Geometry: final body of the model. Coordinates: model frame, mm. A direction names the side the tool comes from. Round coordinates to 2 decimals unless told otherwise and drop trailing zeros. Write each loop counter-clockwise with the first axis right and the second up, starting at its lowest first coordinate (ties: lowest second). Pieces come first, ordered by that corner, then holes. Notation, with made-up numbers: (27, -25) -> (65, -25) arc R36 cw to (65, 9) -> close; hole circle Ø9 at (38, 79). An arc over 180 degrees is marked (long way). Use one line per item in the form item = value. Start each with the question number.
1. Cut plane B-B, the plane y = 0. Return the cut outline in (x, z) (3 decimals).
2. Cut plane C-C, the plane x = 119. Return the cut outline in (y, z) (3 decimals), plus the area to 3 significant figures.
3. Cut plane A-A, the plane z = 18. Return the cut outline in (x, y) (3 decimals).
4. Pin query (flat end, axial travel): pin 1 Ø11.5 at (x, y) = (146.05, 0) entering from -Z. Return the tip coordinate at first contact, or that it passes through.
5. Line query: L1, parallel to X at y = 0, z = 23.55 (3 decimals); L2, parallel to Z at x = 103, y = 7.5 (3 decimals); L3, parallel to Y at x = 84, z = 13 (3 decimals). Output: solid intervals per line, ascending.
6. Cut plane D-D, the plane y = 7. Return the cut outline in (x, z) (3 decimals), plus the area to 3 significant figures.
7. Reachability of faces 4 (the face through (72, 12.7, 13)), 5 (the face through (74, -9.525, 13)) from +Z, -Z, +X, -X, +Y, -Y: full face, straight path, thin tool, end or side. Return the list, or none.
8. Draft query along Z for faces 1 (the face through (74, 0, 3.175)), 2 (the face through (72, 0, 25.4)), 3 (the face through (158.75, 11, 13)). Return one class per face: pulls with the +Z half, pulls with the -Z half, needs draft (parallel to the pull), parting line crosses it, or undercut.
```python
from build123d import *

# Parameters (mm, degrees)
SKETCH1_W           = 171.45
SKETCH1_H           = 25.4
SKETCH1_R           = 9.525
BOSS_EXTRUDE1_DEPTH = 25.4
SKETCH2_W           = 19.05
SKETCH2_H           = 19.05
CUT_EXTRUDE1_DEPTH  = 174.785938729


with BuildPart() as part:
    # Sketch1 → Boss-Extrude1 (new body)
    with BuildSketch(Plane.XY):
        with Locations((73.025, 0)):
            Rectangle(SKETCH1_W, SKETCH1_H)
        Circle(SKETCH1_R, mode=Mode.SUBTRACT)
        with Locations((146.05, 0)):
            Circle(SKETCH1_R, mode=Mode.SUBTRACT)
    extrude(amount=BOSS_EXTRUDE1_DEPTH)

    # Sketch2 → Cut-Extrude1 (cut, through all)
    with BuildSketch(Plane(origin=(158.75, 0, 0), x_dir=(0, 0, -1), z_dir=(1, 0, 0))):
        with Locations((-12.7, 0)):
            Rectangle(SKETCH2_W, SKETCH2_H)
    extrude(amount=-CUT_EXTRUDE1_DEPTH, mode=Mode.SUBTRACT)


solid = part.part
```
Outcome:
q1.outline = (-12.7, 0) -> (-9.525, 0) -> (-9.525, 3.175) -> (-12.7, 3.175) -> close; (-12.7, 22.225) -> (-9.525, 22.225) -> (-9.525, 25.4) -> (-12.7, 25.4) -> close; (9.525, 0) -> (136.525, 0) -> (136.525, 3.175) -> (9.525, 3.175) -> close; (9.525, 22.225) -> (136.525, 22.225) -> (136.525, 25.4) -> (9.525, 25.4) -> close; (155.575, 0) -> (158.75, 0) -> (158.75, 3.175) -> (155.575, 3.175) -> close; (155.575, 22.225) -> (158.75, 22.225) -> (158.75, 25.4) -> (155.575, 25.4) -> close
q2.outline = (-12.7, 0) -> (12.7, 0) -> (12.7, 25.4) -> (-12.7, 25.4) -> close; hole (-9.525, 3.175) -> (9.525, 3.175) -> (9.525, 22.225) -> (-9.525, 22.225) -> close
q2.area = 282 mm^2
q3.outline = (-12.7, -12.7) -> (158.75, -12.7) -> (158.75, -9.525) -> (-12.7, -9.525) -> close; (-12.7, 9.525) -> (158.75, 9.525) -> (158.75, 12.7) -> (-12.7, 12.7) -> close
q4.pin_1 = through
q5.L1 = -12.7 to -9.525, 9.525 to 136.525, 155.575 to 158.75
q5.L2 = 0 to 3.175, 22.225 to 25.4
q5.L3 = -12.7 to -9.525, 9.525 to 12.7
q6.outline = (-12.7, 0) -> (-6.46, 0) -> (-6.46, 3.175) -> (-12.7, 3.175) -> close; (-12.7, 22.225) -> (-6.46, 22.225) -> (-6.46, 25.4) -> (-12.7, 25.4) -> close; (6.46, 0) -> (139.59, 0) -> (139.59, 3.175) -> (6.46, 3.175) -> close; (6.46, 22.225) -> (139.59, 22.225) -> (139.59, 25.4) -> (6.46, 25.4) -> close; (152.51, 0) -> (158.75, 0) -> (158.75, 3.175) -> (152.51, 3.175) -> close; (152.51, 22.225) -> (158.75, 22.225) -> (158.75, 25.4) -> (152.51, 25.4) -> close
q6.area = 925 mm^2
q7.face_4 = +Z, -Z, +X, -X, +Y
q7.face_5 = +X, -X
q8.face_1 = undercut
q8.face_2 = pulls with the +Z half
q8.face_3 = needs draft
